The listing builds one solid part. Answer for the finished solid, in the listing's coordinates (mm). Face numbers are marked on the shaded views. A direction names the side the tool comes from. Give positions to 0.01 mm unless a question says otherwise; leave off trailing zeros. Order: outer loops, then holes, each group sorted by start corner. A loop starts at its lowest first (then second) coordinate and runs counter-clockwise, first axis right, second up. Notation, with made-up numbers: (78, 12) - (126, 12) arc R19 cw to (126, 20) - close; hole circle Ø4 at (-33, 38). An arc over 180 degrees is marked (long way). Answer as CSV lines item,"result". Start each with the question number.
1. Section D-D on x = 26.5 is taken. Give the vertices of the cut face in (y, z), and give its area (3 significant figures).
2. Which of the six approach directions +Z, -Z, +X, -X, +Y, -Y give full straight-line access (tool end or side, diameter ignored) to the marked faces 1 and 2?
3. Section B-B on z = 10.75 is taken. Give the vertices of the cut face in (x, y), and give its area (3 significant figures).
4. Flat-ended cylindrical pins translate along their axes: pin 1 (2 mm diameter, centred on y = 18.5, z = 8.5, fed in from -X); pin 2 (0.9 mm diameter, centred on y = 15.5, z = 1, fed in from +X); pin 3 (3 mm diameter, centred on x = 33, z = 6.5, fed in from +Y); pin 4 (2 mm diameter, centred on x = 29, z = 7.5, fed in from +Y). Find the tip coordinate at first contact, or state that the pin passes through.
5. Section C-C on z = 1.5 is taken. Give the vertices of the cut face in (x, y), and give its area (3 significant figures).
6. Section A-A on y = 23.5 is taken. Give the vertices of the cut face in (x, z), and give its area (3 significant figures).
7. Consider line 1 along X through (y, z) = (2.05, 7.5); line 2 along X through (y, z) = (12, 8); line 3 along Z through (x, y) = (29, 1.6). Determine where each line is inside the solid, lowest interval first. Write a range as [from, to].
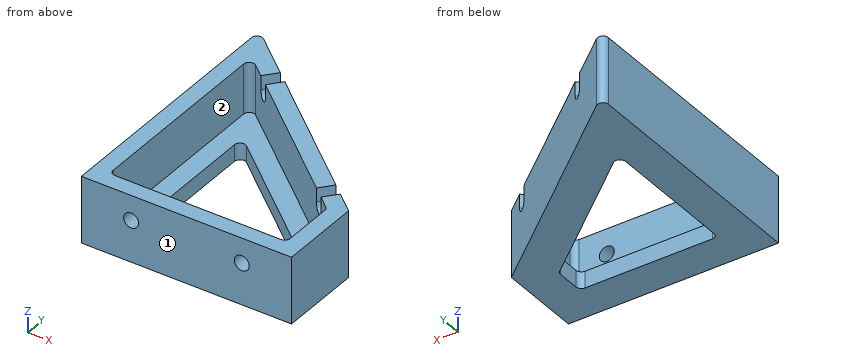
Autodesk Inventor part; units mm, degrees
ref_plane "YZ Plane" through (0, 0, 0) normal (1, 0, 0) x (0, 1, 0)
ref_plane "XZ Plane" through (0, 0, 0) normal (0, 1, 0) x (-1, 0, 0)
ref_plane "XY Plane" through (0, 0, 0) normal (0, 0, 1) x (1, 0, 0)
sketch "Skizze1" plane through (0, 0, 0) normal (0, 0, 1) x (1, 0, 0)
  line L0 (0, 0) -> (0, 46.8858)
  line L1 (0, 46.8858) -> (38, 15)
  line L2 (38, 15) -> (38, 0)
  line L3 (38, 0) -> (0, 0)
  line L4 (6.5, 32.9465) -> (6.5, 6.5)
  line L5 (6.5, 6.5) -> (31.5, 6.5)
  line L6 (31.5, 6.5) -> (31.5, 11.969)
  line L7 (31.5, 11.969) -> (6.5, 32.9465)
  dimension "d0" = 130
  dimension "d1" = 15
  dimension "d2" = 38
  dimension "d3" = 6.5
  dimension "d4" = 6.5
  dimension "d5" = 6.5
  dimension "d6" = 6.5
extrude "Extrusion1" add sketch "Skizze1" along normal blind 12
sketch "Skizze2" plane through (0, 0, 12) normal (0, 0, 1) x (1, 0, 0)
  line L0 (3, 40.4523) -> (3, 3)
  line L1 (3, 3) -> (35, 3)
  line L2 (35, 3) -> (35, 13.6011)
  line L3 (35, 13.6011) -> (3, 40.4523)
  line L4 (0, 0) -> (38, 0)
  line L5 (0, 46.8858) -> (0, 0)
  line L6 (38, 15) -> (0, 46.8858)
  line L7 (38, 0) -> (38, 15)
  dimension "d9" = 3
  dimension "d10" = 3
  dimension "d11" = 3
  dimension "d12" = 3
extrude "Extrusion2" cut sketch "Skizze2" against normal blind 9 contours L3 L2 L1 L0
sketch "Skizze3" plane through (3, 3, 12) normal (0, 1, 0) x (1, 0, 0)
  line L0 (-3, 0) -> (-3, 12)
  line L1 (-3, 12) -> (35, 12)
  line L2 (35, 12) -> (35, 0)
  line L3 (35, 0) -> (32, 0)
  line L4 (32, 0) -> (0, 0)
  line L5 (0, 0) -> (-3, 0)
  line L6 (32, 0) -> (32, 9)
  line L7 (32, 9) -> (0, 9)
  line L8 (0, 9) -> (0, 0)
  line L9 (0, 0) -> (0, 9)
  line L10 (32, 0) -> (32, 9)
  line L11 (32, 4.5) -> (0, 4.5)
  point P0 (6, 4.5)
  point P1 (26, 4.5)
  dimension "d15" = 6
  dimension "d17" = 6
hole "Bohrung1" at (9, 3, 7.5) at (29, 3, 7.5) direction (0, -1, 0) diameter 2.7 depth 8 tip angle 118
fillet "Rundung1" radius 1 9 edges at (35, 13.6011, 7.5) (31.5, 11.969, 1.5) (31.5, 6.5, 1.5) (35, 3, 7.5) (6.5, 6.5, 1.5) (3, 3, 7.5) (6.5, 32.9465, 1.5) (3, 40.4523, 7.5) (0, 46.8858, 6)
sketch "Skizze4" plane through (4.6428, 39.0738, 3) normal (-0.6427876, -0.7660444, 0) x (0.7660444, -0.6427876, 0)
  line L0 (-6.0607, 9) -> (0, 9)
  line L1 (0, 9) -> (39.1622, 9)
  line L2 (39.1622, 9) -> (43.5447, 9)
  line L3 (43.5447, 9) -> (43.5447, -3)
  line L4 (43.5447, -3) -> (-6.0607, -3)
  line L5 (-6.0607, -3) -> (-6.0607, 9)
  line L6 (0, 0) -> (0, 9)
  line L7 (0, 0) -> (39.1622, 0)
  line L8 (39.1622, 0) -> (39.1622, 9)
  point P0 (21.5596, -3)
  point P1 (35.1622, 6.5)
  point P2 (4.1622, 6.5)
  point P3 (35.1622, 6.5)
  dimension "d26" = 2.5
  dimension "d27" = 4
  dimension "d28" = 2.5
  dimension "d29" = 35
  dimension "d30" = 4.1622
hole "Bohrung2" at (31.5786, 16.472, 9.5) at (7.8312, 36.3984, 9.5) direction (0.6427876, 0.7660444, 0) diameter 2.5 depth 8 tip angle 118
sketch "Skizze5" plane through (38, 15, 12) normal (0.6427876, 0.7660444, 0) x (0.7660444, -0.6427876, 0)
  circle A0 centre (-5.8652, 2.5) radius 1.25
  line L0 (-4.6152, 2.5) -> (-4.6152, 0)
  line L1 (-19.4679, 0) -> (9.6418, 0)
  line L2 (-7.1152, 2.5) -> (-7.1152, 0)
  circle A1 centre (-36.8652, 2.5) radius 1.25
  line L3 (-35.6152, 2.5) -> (-35.6152, 0)
  line L4 (-41.0274, 0) -> (-1.8652, 0)
  line L5 (-38.1152, 2.5) -> (-38.1152, 0)
  point P0 (-19.4679, 12)
extrude "Extrusion3" cut sketch "Skizze5" against normal blind 4.5 contours L0 L1 L2 A0 | L3 L4 L5 A1
properties part number "lcd_halterung_162C_links"
Checks:
1,outline,"(0, 0) - (6.5, 0) - (6.5, 3) - (3, 3) - (3, 12) - (0, 12) - close; (16.16, 0) - (24.65, 0) - (24.65, 12) - (20.73, 12) - (20.73, 3) - (16.16, 3) - close"
1,area,"107 mm²"
2,face 1,"+Z, -Z, +X, -X, -Y"
2,face 2,"+Z"
3,outline,"(0, 0) - (38, 0) - (38, 15) - (34.46, 17.97) - (32.54, 15.67) - (34.64, 13.9) arc R1 cw to (35, 13.13) - (35, 4) arc R1 cw to (34, 3) - (4, 3) arc R1 cw to (3, 4) - (3, 38.31) arc R1 cw to (4.64, 39.07) - (6.87, 37.2) - (8.8, 39.5) - (1.64, 45.51) arc R1 ccw to (0, 44.74) - close; (8.79, 35.59) - (30.62, 17.28) - (32.55, 19.57) - (10.72, 37.89) - close"
3,area,"392 mm²"
4,pin 1,"stops at x = 0"
4,pin 2,"stops at x = 37.94"
4,pin 3,"stops at y = 20.45"
4,pin 4,"stops at y = 23.39"
5,outline,"(0, 0) - (38, 0) - (38, 15) - (1.64, 45.51) arc R1 ccw to (0, 44.74) - close; hole (6.5, 7.5) arc R1 ccw to (7.5, 6.5) - (30.5, 6.5) arc R1 ccw to (31.5, 7.5) - (31.5, 11.5) arc R1 ccw to (31.14, 12.27) - (8.14, 31.57) arc R1 ccw to (6.5, 30.8) - close"
5,area,"777 mm²"
6,outline,"(0, 0) - (6.5, 0) - (6.5, 3) - (3, 3) - (3, 12) - (0, 12) - close; (17.76, 0) - (27.87, 0) - (27.87, 12) - (23.2, 12) - (23.2, 3) - (17.76, 3) - close"
6,area,"119 mm²"
7,line 1,"x = [0, 7.65], [10.35, 27.65], [30.35, 38]"
7,line 2,"x = [0, 3], [35, 38]"
7,line 3,"z = [0, 6.15], [8.85, 12]"
